Input: part model. Units: mm. Frame: model coordinates. Face numbers are marked on the shaded views. A direction names the side the tool comes from. Round coordinates to 2 decimals unless told otherwise and drop trailing zeros. Write each loop counter-clockwise with the first axis right and the second up, starting at its lowest first coordinate (ties: lowest second). Pieces come first, ordered by that corner, then holes. Notation, with made-up numbers: (51, -29.75) -> (100, -29.75) arc R21 cw to (100, -11.75) -> close; hole circle Ø2 at (-23, -35.75). An arc over 180 degrees is marked (long way). Write item = value, one per line.
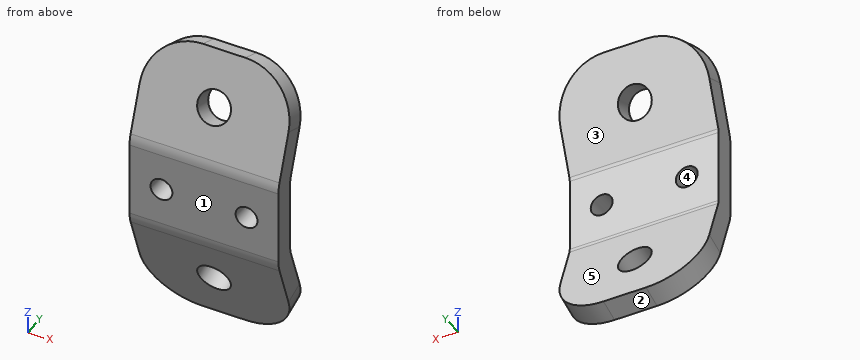
```python
from build123d import *

# Parameters (mm, degrees)
BASE_FLANGE1_DEPTH = 22.225
FILLET1_R          = 15.875
SKETCH6_R          = 4.9657
CUT_EXTRUDE1_DEPTH = 7.62
SKETCH7_R          = 4.9657
CUT_EXTRUDE2_DEPTH = 7.62
SKETCH8_R          = 3.2639
CUT_EXTRUDE3_DEPTH = 7.62


# Sheet-metal steps are written as plain solids
with BuildPart() as part:
    # Sketch1 → Base-Flange1 (new, symmetric)
    with BuildSketch(Plane(origin=(0, 0, 0), x_dir=(0, 0, -1), z_dir=(1, 0, 0))):
        with BuildLine():
            Line((-42.53524071, 10.859139551), (-14.278227374, 0.574427787))
            ThreePointArc((-14.278227374, 0.574427787), (-12.674484401, 0.144706153), (-11.020485509, 0))
            Line((-11.020485509, 0), (11.020485509, 0))
            ThreePointArc((11.020485509, 0), (12.674484401, 0.144706153), (14.278227374, 0.574427787))
            Line((14.278227374, 0.574427787), (42.53524071, 10.859139551))
            Line((42.53524071, 10.859139551), (40.3634128, 16.826187693))
            Line((40.3634128, 16.826187693), (12.106399464, 6.541475929))
            ThreePointArc((12.106399464, 6.541475929), (11.571818473, 6.398235384), (11.020485509, 6.35))
            Line((11.020485509, 6.35), (-11.020485509, 6.35))
            ThreePointArc((-11.020485509, 6.35), (-11.571818473, 6.398235384), (-12.106399464, 6.541475929))
            Line((-12.106399464, 6.541475929), (-40.3634128, 16.826187693))
            Line((-40.3634128, 16.826187693), (-42.53524071, 10.859139551))
        make_face()
    extrude(amount=BASE_FLANGE1_DEPTH, both=True)

    # Fillet1
    fillet1_edges = [part.edges().sort_by_distance(p)[0] for p in [
        (-22.225, 13.842663622, -41.449326755),
        (-22.225, 13.842663622, 41.449326755),
        (22.225, 13.842663622, -41.449326755),
        (22.225, 13.842663622, 41.449326755),
    ]]
    fillet(fillet1_edges, radius=FILLET1_R)

    # Sketch6 → Cut-Extrude1 (cut)
    with BuildSketch(Plane(origin=(0, -4.081701322, -1.485617786), x_dir=(1, 0, 0), z_dir=(0, -0.9396926207859082, -0.34202014332566943))):
        with Locations(Location((0, -27.809096284, 0), (0, 0, 270))):
            Circle(SKETCH6_R)
    extrude(amount=-CUT_EXTRUDE1_DEPTH, mode=Mode.SUBTRACT)

    # Sketch7 → Cut-Extrude2 (cut)
    with BuildSketch(Plane(origin=(0, -4.081701322, 1.485617786), x_dir=(1, 0, 0), z_dir=(0, -0.9396926207859082, 0.34202014332566943))):
        with Locations(Location((0, 27.809096284, 0), (0, 0, 270))):
            Circle(SKETCH7_R)
    extrude(amount=-CUT_EXTRUDE2_DEPTH, mode=Mode.SUBTRACT)

    # Sketch8 → Cut-Extrude3 (cut)
    with BuildSketch(Plane.XZ):
        with Locations(Location((-12.7, 0, 0), (0, 0, 270))):
            Circle(SKETCH8_R)
        with Locations(Location((12.7, 0, 0), (0, 0, 270))):
            Circle(SKETCH8_R)
    extrude(amount=-CUT_EXTRUDE3_DEPTH, mode=Mode.SUBTRACT)


solid = part.part
```
1) Cut plane A-A (z = 0). Return the cut outline in (x, y) (3 decimals).
Solutions:
outline = (-22.225, 0) -> (-15.964, 0) -> (-15.964, 6.35) -> (-22.225, 6.35) -> close; (-9.436, 0) -> (9.436, 0) -> (9.436, 6.35) -> (-9.436, 6.35) -> close; (15.964, 0) -> (22.225, 0) -> (22.225, 6.35) -> (15.964, 6.35) -> close
2) Draft query along Z for the marked faces 1, 2 and 3. Return one class per face: +Z half, -Z half, draft (parallel to the pull), parting line (faces both ways), or undercut.
Solutions:
face_1 = draft
face_2 = -Z half
face_3 = undercut
3) Cut plane C-C (y = 2.25). Return the cut outline in (x, z) (3 decimals), and give its area (3 significant figures).
Solutions:
outline = (-22.225, -18.882) -> (22.225, -18.882) -> (22.225, 18.882) -> (-22.225, 18.882) -> close; hole circle Ø6.528 at (-12.7, 0); hole circle Ø6.528 at (12.7, 0)
area = 1,610 mm^2
4) Line query: L1, parallel to X at y = 3.5, z = 0 (3 decimals); L2, parallel to Y at x = 10.5, z = -8; L3, parallel to Y at x = 15.5, z = 20. Output: solid intervals per line, ascending. Write a range as from..to.
Solutions:
L1 = -22.225..-15.964, -9.436..9.436, 15.964..22.225
L2 = 0..6.35
L3 = 2.66..9.41
5) Access query for the marked faces 4 and 5. Directions: +Z, -Z, +X, -X, +Y, -Y. A direction counts if a zero-diameter tool reaches every point of the face in a straight line with its end or side. Return the directions, or none.
Solutions:
face_4 = +Y, -Y
face_5 = +X, -X, +Y
6) First-contact query: P1, Ø5, axis at y = 3.5, z = -30, coming from the +X side; P2, Ø4, axis at x = 14.5, z = -27.5, coming from the +Y side; P3, Ø8, axis at y = 7.5, z = 33, coming from the -X side; P4, Ø2, axis at x = -8, z = -6, coming from the +Y side. Flat tips, straight axial feed; report the tip coordinate or a pass-through.
Solutions:
P1 = through
P2 = 12.87
P3 = -22.13
P4 = 6.35
7) Cut plane D-D (x = -3). Return the cut outline in (y, z) (3 decimals).
Solutions:
outline = (0, -11.02) arc R9.525 ccw to (0.574, -14.278) -> (4.076, -23.899) -> (10.043, -21.727) -> (6.541, -12.106) arc R3.175 cw to (6.35, -11.02) -> (6.35, 11.02) arc R3.175 cw to (6.541, 12.106) -> (10.043, 21.727) -> (4.076, 23.899) -> (0.574, 14.278) arc R9.525 ccw to (0, 11.02) -> close; (6.783, -31.336) -> (10.859, -42.535) -> (16.826, -40.363) -> (12.75, -29.164) -> close; (6.783, 31.336) -> (12.75, 29.164) -> (16.826, 40.363) -> (10.859, 42.535) -> close
8) Cut plane B-B (x = 11). Return the cut outline in (y, z) (3 decimals).
Solutions:
outline = (0, -11.02) arc R9.525 ccw to (0.574, -14.278) -> (10.621, -41.881) -> (16.588, -39.709) -> (6.541, -12.106) arc R3.175 cw to (6.35, -11.02) -> (6.35, -2.786) -> (0, -2.786) -> close; (0, 2.786) -> (6.35, 2.786) -> (6.35, 11.02) arc R3.175 cw to (6.541, 12.106) -> (16.588, 39.709) -> (10.621, 41.881) -> (0.574, 14.278) arc R9.525 ccw to (0, 11.02) -> close
